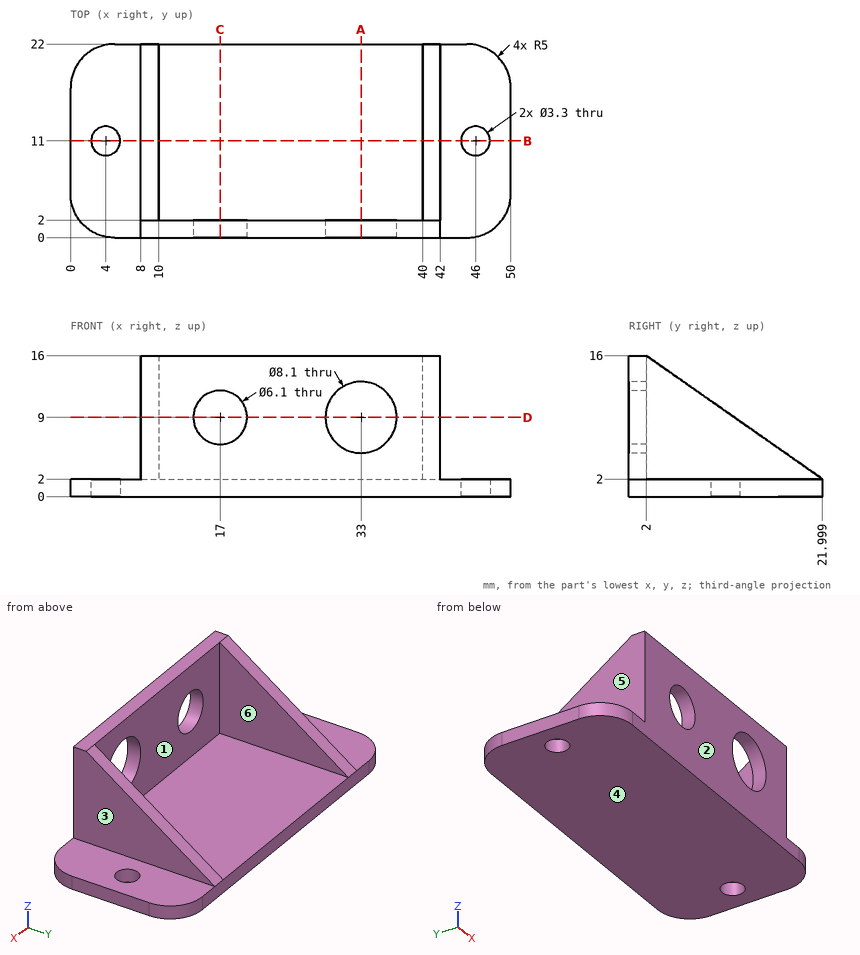
Input: dimensioned drawing with shaded views. Units: mm. Origin: part minimum x, y, z. A direction names the side the tool comes from. Give positions to 0.01 mm unless a question says otherwise; leave off trailing zeros. Order: outer loops, then holes, each group sorted by start corner. A loop starts at its lowest first (then second) coordinate and runs counter-clockwise, first axis right, second up.
(1) Section query B-B (y = 11). Return the cut outline in (x, z), plus the area to 3 significant figures.
(2) Section query A-A (x = 33). Return the cut outline in (y, z), plus the area to 3 significant figures.
(3) Section query D-D (z = 9). Return the cut outline in (x, y).
(4) Contact query for flat-ended pins moving along their axis: P1, Ø1.5, axis at x = 29.5, y = 13, coming from the +Z side; P2, Ø6, axis at y = 10.5, z = 12, coming from the +X side; P3, Ø5, axis at y = 9.5, z = 3, coming from the -X side; P4, Ø5, axis at x = 33, z = 9, coming from the +Y side. Output: stop coordinate, or through.
(5) Pull-direction query (X, two-part tool) for the marked faces 3, 4, 5 and 6; classes: +X half, -X half, draft (parallel to the pull), parting line (faces both ways), or undercut.
(6) Access query for the marked faces 1 and 2. Directions: +Z, -Z, +X, -X, +Y, -Y. A direction counts if a zero-diameter tool reaches every point of the face in a straight line with its end or side. Return the directions, or none.
(7) Material intervals for line 1 along X through (y, z) = (3.5, 8.25); line 2 along Z through (x, y) = (33, 0.4); line 3 along Z through (x, y) = (17, 0.7), sorted ascending.
(8) Section query C-C (x = 17). Return the cut outline in (y, z).
Outcome:
1. outline: (0, 0) - (2.35, 0) - (2.35, 2) - (0, 2) - close; (5.65, 0) - (44.35, 0) - (44.35, 2) - (42, 2) - (42, 9.7) - (40, 9.7) - (40, 2) - (10, 2) - (10, 9.7) - (8, 9.7) - (8, 2) - (5.65, 2) - close; (47.65, 0) - (50, 0) - (50, 2) - (47.65, 2) - close
1. area: 118 mm2
2. outline: (0, 0) - (22, 0) - (22, 2) - (2, 2) - (2, 4.95) - (0, 4.95) - close; (0, 13.05) - (2, 13.05) - (2, 16) - (0, 16) - close
2. area: 55.8 mm2
3. outline: (8, 0) - (13.95, 0) - (13.95, 2) - (10, 2) - (10, 12) - (8, 12) - close; (20.05, 0) - (28.95, 0) - (28.95, 2) - (20.05, 2) - close; (37.05, 0) - (42, 0) - (42, 12) - (40, 12) - (40, 2) - (37.05, 2) - close
4. P1: stops at z = 2
4. P2: stops at x = 42
4. P3: stops at x = 0
4. P4: passes through
5. face 3: +X half
5. face 4: draft
5. face 5: -X half
5. face 6: undercut
6. face 1: +Z, +Y
6. face 2: +Z, -Z, +X, -X, -Y
7. line 1: x = 8 to 10, 40 to 42
7. line 2: z = 0 to 4.95, 13.05 to 16
7. line 3: z = 0 to 5.95, 12.05 to 16
8. outline: (0, 0) - (22, 0) - (22, 2) - (2, 2) - (2, 5.95) - (0, 5.95) - close; (0, 12.05) - (2, 12.05) - (2, 16) - (0, 16) - close
